from build123d import *

# Parameters (mm, degrees)
SKETCH1_W           = 39.69
SKETCH1_H           = 3.175
BOSS_EXTRUDE1_DEPTH = 12.7
SKETCH3_W           = 6.35
SKETCH3_H           = 0.4
SKETCH3_W_2         = 0.4
SKETCH3_H_2         = 6.35
CUT_EXTRUDE7_DEPTH  = 3.175
CUT_EXTRUDE8_DEPTH  = 3.175


with BuildPart() as part:
    # Sketch1 → Boss-Extrude1 (new body)
    with BuildSketch(Plane(origin=(0, 0, 0), x_dir=(1, 0, 0), z_dir=(0, 1, 0))):
        Rectangle(SKETCH1_W, SKETCH1_H)
    extrude(amount=BOSS_EXTRUDE1_DEPTH)

    # Sketch3 → Cut-Extrude7 (cut)
    with BuildSketch(Plane.XY.offset(1.5875)):
        with Locations((-0.043891751, 6.35)):
            Rectangle(SKETCH3_W, SKETCH3_H)
        with Locations((-0.043891751, 6.35)):
            Rectangle(SKETCH3_W_2, SKETCH3_H_2)
    extrude(amount=-CUT_EXTRUDE7_DEPTH, mode=Mode.SUBTRACT)

    # Sketch6 → Cut-Extrude8 (cut)
    with BuildSketch(Plane.XY.offset(1.5875)):
        Polygon((-3.218891751, 9.525), (-3.218891751, 12.7), (-19.845, 12.7), (-19.845, 3.175), align=None)
        Polygon((19.845, 12.7), (3.131108249, 12.7), (3.131108249, 9.525), (19.845, 3.175), align=None)
    extrude(amount=-CUT_EXTRUDE8_DEPTH, mode=Mode.SUBTRACT)


solid = part.part
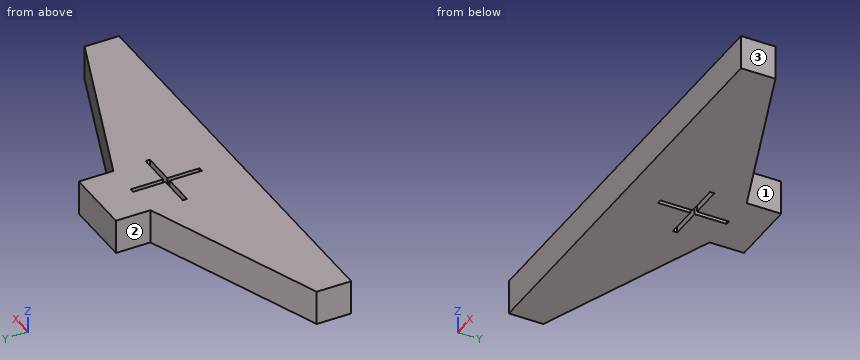
Verification items for the finished model (mm, model axes). Face numbers are marked on the shaded views. A direction names the side the tool comes from. Give positions to 0.01 mm unless a question says otherwise; leave off trailing zeros. Loops run counter-clockwise (first coordinate to the right, second up) from the corner with the lowest first, then second, coordinate; pieces in that order, holes last.
1. Cross-section at B-B on z = 1.1. Record the cut outline in (x, y) (3 decimals).
Derived:
outline: (-19.845, 0) - (19.845, 0) - (19.845, 3.175) - (3.131, 9.525) - (3.131, 12.7) - (-3.219, 12.7) - (-3.219, 9.525) - (-19.845, 3.175) - close; hole (-3.219, 6.15) - (-0.244, 6.15) - (-0.244, 3.175) - (0.156, 3.175) - (0.156, 6.15) - (3.131, 6.15) - (3.131, 6.55) - (0.156, 6.55) - (0.156, 9.525) - (-0.244, 9.525) - (-0.244, 6.55) - (-3.219, 6.55) - close
2. Cross-section at C-C on y = 5.75. Record the cut outline in (x, z), and give its area (3 significant figures).
Derived:
outline: (-13.1, -1.59) - (-0.24, -1.59) - (-0.24, 1.59) - (-13.1, 1.59) - close; (0.16, -1.59) - (13.07, -1.59) - (13.07, 1.59) - (0.16, 1.59) - close
area: 81.8 mm2
3. Go/stop test with flat-tipped pins: P1, Ø1.6, axis at y = 11.5, z = -0.5, coming from the +X side; P2, Ø1.6, axis at y = 11, z = -0.5, coming from the -X side. Record where each tip stops, or that it passes through.
Derived:
P1: stops at x = 3.13
P2: stops at x = -3.22
4. Cross-section at A-A on x = 2. Record the cut outline in (y, z).
Derived:
outline: (0, -1.59) - (6.15, -1.59) - (6.15, 1.59) - (0, 1.59) - close; (6.55, -1.59) - (12.7, -1.59) - (12.7, 1.59) - (6.55, 1.59) - close
5. Cross-section at D-D on y = 10.75. Record the cut outline in (x, z).
Derived:
outline: (-3.22, -1.59) - (3.13, -1.59) - (3.13, 1.59) - (-3.22, 1.59) - close
6. Tool access check on the marked faces 1, 2 and 3. Record the directions out of +Z, -Z, +X, -X, +Y, -Y that give a thin tool (end or side, any length) a straight path to the whole face; none if there is none.
Derived:
face 1: +Z, -Z, +X, +Y
face 2: +Z, -Z, -X, +Y
face 3: +Z, -Z, +X, +Y, -Y
7. Material ranges on probe 1 along Y at (x, z) = (-0.5, -0.65); probe 2 along Y at (x, z) = (0, -0.1) (3 decimals); probe 3 along X at (y, z) = (10.5, -0.85), recorded low to high.
Derived:
probe 1: y = 0 to 6.15, 6.55 to 12.7
probe 2: y = 0 to 3.175, 9.525 to 12.7
probe 3: x = -3.22 to 3.13
